from build123d import *

# Parameters (mm, degrees)
PAD003_DEPTH = 2
SKETCH013_W  = 54
SKETCH013_H  = 54
SKETCH013_R  = 1.75
PAD004_DEPTH = 2


with BuildPart() as part:
    # Sketch016 → Pad003 (new body)
    with BuildSketch(Plane.XY.offset(7)):
        with BuildLine():
            ThreePointArc((26, 0), (24.828437, 2.828417), (22.000028, 4))
            Line((22.000028, 4), (0, 4))
            ThreePointArc((0, 4), (-2.828427, 2.828427), (-4, 0))
            Line((-4, 0), (-4, -22.000028))
            ThreePointArc((-4, -22.000028), (-2.828417, -24.828437), (0, -26))
            Line((0, -26), (22.000028, -26))
            ThreePointArc((22.000028, -26), (24.828427, -24.828427), (26, -22.000028))
            Line((26, -22.000028), (26, 0))
        make_face()
    extrude(amount=PAD003_DEPTH)

    # Sketch014 → AdditiveLoft section 0
    with BuildSketch(Plane.XY.offset(12)):
        with BuildLine():
            ThreePointArc((23.2, 0), (22.848528, 0.848529), (21.999999, 1.2))
            Line((21.999999, 1.2), (0, 1.2))
            ThreePointArc((0, 1.2), (-0.848528, 0.848528), (-1.2, 0))
            Line((-1.2, 0), (-1.2, -21.999999))
            ThreePointArc((-1.2, -21.999999), (-0.848529, -22.848528), (0, -23.2))
            Line((0, -23.2), (21.999999, -23.2))
            ThreePointArc((21.999999, -23.2), (22.848528, -22.848528), (23.2, -21.999999))
            Line((23.2, -21.999999), (23.2, 0))
        make_face()
    # Sketch015 → AdditiveLoft section 1
    with BuildSketch(Plane.XY.offset(7)):
        with BuildLine():
            ThreePointArc((23.2, 0), (22.848528, 0.848529), (21.999999, 1.2))
            Line((21.999999, 1.2), (0, 1.2))
            ThreePointArc((0, 1.2), (-0.848528, 0.848528), (-1.2, 0))
            Line((-1.2, 0), (-1.2, -21.999999))
            ThreePointArc((-1.2, -21.999999), (-0.848529, -22.848528), (0, -23.2))
            Line((0, -23.2), (21.999999, -23.2))
            ThreePointArc((21.999999, -23.2), (22.848528, -22.848528), (23.2, -21.999999))
            Line((23.2, -21.999999), (23.2, 0))
        make_face()
    loft()

    # Sketch013 → Pad004 (join)
    with BuildSketch(Plane.XY.offset(12)):
        with Locations((11, -11)):
            Rectangle(SKETCH013_W, SKETCH013_H)
        with Locations((-12, 12)):
            Circle(SKETCH013_R, mode=Mode.SUBTRACT)
        with Locations((34, 12)):
            Circle(SKETCH013_R, mode=Mode.SUBTRACT)
        with Locations((34, -34)):
            Circle(SKETCH013_R, mode=Mode.SUBTRACT)
        with Locations((-12, -34)):
            Circle(SKETCH013_R, mode=Mode.SUBTRACT)
        with Locations((34, -11)):
            Circle(SKETCH013_R, mode=Mode.SUBTRACT)
        with Locations((34, 0.5)):
            Circle(SKETCH013_R, mode=Mode.SUBTRACT)
        with Locations((34, -22.5)):
            Circle(SKETCH013_R, mode=Mode.SUBTRACT)
        with Locations((22.5, -34)):
            Circle(SKETCH013_R, mode=Mode.SUBTRACT)
        with Locations((11, -34)):
            Circle(SKETCH013_R, mode=Mode.SUBTRACT)
        with Locations((-0.5, -34)):
            Circle(SKETCH013_R, mode=Mode.SUBTRACT)
        with Locations((-12, -22.5)):
            Circle(SKETCH013_R, mode=Mode.SUBTRACT)
        with Locations((-12, -11)):
            Circle(SKETCH013_R, mode=Mode.SUBTRACT)
        with Locations((-12, 0.5)):
            Circle(SKETCH013_R, mode=Mode.SUBTRACT)
        with Locations((11, 12)):
            Circle(SKETCH013_R, mode=Mode.SUBTRACT)
        with Locations((22.5, 12)):
            Circle(SKETCH013_R, mode=Mode.SUBTRACT)
        with Locations((-0.5, 12)):
            Circle(SKETCH013_R, mode=Mode.SUBTRACT)
    extrude(amount=PAD004_DEPTH)


solid = part.part
Source: CAD feature listing. Evaluate the final solid. Frame: model axes, mm. A direction names the side the tool comes from. Give positions to 0.01 mm unless a question says otherwise; leave off trailing zeros. Write each loop counter-clockwise with the first axis right and the second up, starting at its lowest first coordinate (ties: lowest second). Pieces come first, ordered by that corner, then holes. Notation, with made-up numbers: (26, 36) - (71, 36) arc R32 ccw to (71, 71) - close; hole circle Ø4 at (58, 20.25). An arc over 180 degrees is marked (long way). Write item = value, one per line. Start each with the question number.
Q1. Cut plane C-C, the plane x = -12. Return loops of the section in (y, z).
Q2. Cut plane B-B, the plane z = 13.25. Give the number of separate pieces and of enclosed holes in the cut face, then the cut area to 3 significant figures.
Q3. Material intervals for probe 1 along Y at (x, z) = (-12, 12.95); probe 2 along Y at (x, z) = (11, 13.35); probe 3 along Z at (x, y) = (13.5, 3.5), sorted ascending.
Q4. Cut plane A-A, the plane x = 11. Return loops of the section in (y, z).
Q5. Cut plane D-D, the plane y = -29. Return loops of the section in (x, z), then the cut area to 3 significant figures.
Q6. Draft query along Y for faces 1 (the flat face through (11, -38, 13)), 2 (the flat face through (-16, -11, 13)), 3 (the cylindrical face through (-10.331, 1.026, 12.986)), 4 (the cylindrical face through (12.669, 12.526, 12.986)). Return one class per face: +Y half, -Y half, draft (parallel to the pull), parting line (faces both ways), or undercut.
Q7. Reachability of faces 5 (the cylindrical face through (22.839, -22.858, 10.479)), 6 (the flat face through (23.2, -11, 10)), 7 (the flat face through (26, -11, 8)) from +Z, -Z, +X, -X, +Y, -Y: full face, straight path, thin tool, end or side. Return the list, or none.
Q8. Pin query (flat end, axial travel): pin 1 Ø3.5 at (y, z) = (-7, 10.5) entering from +X; pin 2 Ø0.6 at (y, z) = (-7, 8.5) entering from -X; pin 3 Ø2.5 at (x, z) = (13.5, 10.5) entering from -Y; pin 4 Ø0.6 at (x, z) = (6.5, 8) entering from +Y. Return the tip coordinate at first contact, or that it passes through.
Computed values:
q1.outline = (-38, 12) - (-35.75, 12) - (-35.75, 14) - (-38, 14) - close; (-32.25, 12) - (-24.25, 12) - (-24.25, 14) - (-32.25, 14) - close; (-20.75, 12) - (-12.75, 12) - (-12.75, 14) - (-20.75, 14) - close; (-9.25, 12) - (-1.25, 12) - (-1.25, 14) - (-9.25, 14) - close; (2.25, 12) - (10.25, 12) - (10.25, 14) - (2.25, 14) - close; (13.75, 12) - (16, 12) - (16, 14) - (13.75, 14) - close
q2.separate_pieces = 1
q2.enclosed_holes = 16
q2.area = 2,760 mm²
q3.probe_1 = -38 to -35.75, -32.25 to -24.25, -20.75 to -12.75, -9.25 to -1.25, 2.25 to 10.25, 13.75 to 16
q3.probe_2 = -38 to -35.75, -32.25 to 10.25, 13.75 to 16
q3.probe_3 = 7 to 9, 12 to 14
q4.outline = (-38, 12) - (-35.75, 12) - (-35.75, 14) - (-38, 14) - close; (-32.25, 12) - (-23.2, 12) - (-23.2, 9) - (-26, 9) - (-26, 7) - (4, 7) - (4, 9) - (1.2, 9) - (1.2, 12) - (10.25, 12) - (10.25, 14) - (-32.25, 14) - close; (13.75, 12) - (16, 12) - (16, 14) - (13.75, 14) - close
q5.outline = (-16, 12) - (38, 12) - (38, 14) - (-16, 14) - close
q5.area = 108 mm²
q6.face_1 = -Y half
q6.face_2 = draft
q6.face_3 = undercut
q6.face_4 = undercut
q7.face_5 = +X, -Y
q7.face_6 = +X, +Y, -Y
q7.face_7 = -Z, +X, +Y, -Y
q8.pin_1 = 38
q8.pin_2 = -4
q8.pin_3 = -23.2
q8.pin_4 = 4
